Part model, mm, in its own coordinate system. A direction names the side the tool comes from. Give positions to 0.01 mm unless a question says otherwise; leave off trailing zeros. Order: outer loops, then holes, each group sorted by start corner. A loop starts at its lowest first (then second) coordinate and runs counter-clockwise, first axis right, second up.
from build123d import *

# Parameters (mm, degrees)
CROQUIS2_R                          = 7
SALIENTE_EXTRUIR1_DEPTH             = 3
CROQUIS3_R                          = 1.5
SALIENTE_EXTRUIR2_DEPTH             = 6
DI_METRO_DE_TALADRO_3_2_3_2_1_D     = 3.2
DI_METRO_DE_TALADRO_3_2_3_2_1_DEPTH = 10
DI_METRO_DE_TALADRO_4_2_4_2_1_D     = 4.2
DI_METRO_DE_TALADRO_4_2_4_2_1_DEPTH = 12
CHAFL_N1_SIZE                       = 18
CHAFL_N1_SIZE2                      = 4


with BuildPart() as part:
    # Croquis1 → Revolución1 (revolve)
    with BuildSketch(Plane.XY, mode=Mode.PRIVATE) as revoluci_n1_sk:
        with BuildLine():
            Line((34, 38.5), (0, 38.5))
            Line((0, 38.5), (0, 0))
            Line((0, 0), (46, 0))
            Line((46, 0), (46, 30))
            ThreePointArc((46, 30), (41.352720585, 36.159723179), (34, 38.5))
        make_face()
    revolve(revoluci_n1_sk.sketch.rotate(Axis((0, 38.5, 0), (0, -1, 0)), 270), axis=Axis((0, 38.5, 0), (0, -1, 0)))

    # Croquis2 → Saliente-Extruir1 (add)
    with BuildSketch(Plane.XZ):
        with Locations(Location((0, 0, 0), (0, 0, 270))):
            Circle(CROQUIS2_R)
    extrude(amount=SALIENTE_EXTRUIR1_DEPTH)

    # Croquis3 → Saliente-Extruir2 (add)
    with BuildSketch(Plane(origin=(0, 38.5, 0), x_dir=(-1, 0, 0), z_dir=(0, 1, 0))):
        with Locations(Location((0, 0, 0), (0, 0, 90))):
            Circle(CROQUIS3_R)
    extrude(amount=SALIENTE_EXTRUIR2_DEPTH)

    # Diámetro de taladro Ø3.2 (3.2)1
    with Locations(Plane(origin=(0, 38.5, 0), x_dir=(1, 0, 0), z_dir=(0, 1, 0))):
        with Locations((0, 15.5), (-15.5, 0), (15.5, 0), (0, -15.5)):
            Hole(DI_METRO_DE_TALADRO_3_2_3_2_1_D / 2, depth=DI_METRO_DE_TALADRO_3_2_3_2_1_DEPTH)

    # Diámetro de taladro Ø4.2 (4.2)1
    with Locations(Plane(origin=(0, 0, 0), x_dir=(-1, 0, 0), z_dir=(0, -1, 0))):
        with Locations((0, -20), (20, 0), (-20, 0), (0, 20)):
            Hole(DI_METRO_DE_TALADRO_4_2_4_2_1_D / 2, depth=DI_METRO_DE_TALADRO_4_2_4_2_1_DEPTH)

    # Chaflán1
    chafl_n1_edges = [part.edges().sort_by_distance(p)[0] for p in [
        (0, 0, 46),
    ]]
    chafl_n1_side = [part.faces().sort_by_distance(p)[0] for p in [
        (0, 0, 44.698923523),
    ]]
    chamfer(chafl_n1_edges, length=CHAFL_N1_SIZE, length2=CHAFL_N1_SIZE2, reference=chafl_n1_side[0])


solid = part.part
Item 1: Drop flat-ended pins along their axis: P1, Ø2.5, axis at x = 15, z = 0, coming from the +Y side; P2, Ø5, axis at x = -25.5, y = 37, coming from the +Z side; P3, Ø4, axis at y = 20.5, z = -15, coming from the +X side. Give the stop position or say it passes through.
Item 2: Drill centre lines: probe 1 along Y at (x, z) = (-9.5, -15.5); probe 2 along Z at (x, y) = (20, 6); probe 3 along X at (y, z) = (35, -15). Where is each one in solid material? Low to high.
Item 3: Band-saw the part on D-D on y = 24. List the corners of the cut face in (x, z), plus the area to 3 significant figures.
Item 4: Which spindle directions (+Z, -Z, +X, -X, +Y, -Y) get a long thin tool onto all of the face, cutting with end or side? Do faces 5 (the face through (0, 44.5, 0)), 6 (the face through (17.1, 33.43, -0.07)), 7 (the face through (-17.997, 6.084, -0.631)). Say none if no direction does.
Item 5: Band-saw the part on B-B on y = 41.5. List the corners of the cut face in (x, z).
Item 6: Band-saw the part on C-C on y = 34. List the corners of the cut face in (x, z), plus the area to 3 significant figures.
Item 7: Pull direction X, two halves, no side cores. Call faces 1 (the face through (22.003, 6.084, -0.631)), 2 (the face through (0, -3, 0)), 3 (the face through (1.13, 6.08, 18.23)), 4 (the face through (-28.43, 0.25, 6.31)): released by +X, released by -X, zero draft, split by the parting line, or undercut.
Item 8: Band-saw the part on A-A on y = 8. List the corners of the cut face in (x, z).
Working result:
1. P1: stops at y = 38.5
1. P2: stops at z = 35.43
1. P3: stops at x = 44.12
2. probe 1: y = 0 to 38.5
2. probe 2: z = -41.42 to -2.1, 2.1 to 41.42
2. probe 3: x = -40.05 to -1.52, 1.52 to 40.05
3. outline: circle Ø92 at (0, 0)
3. area: 6,650 mm2
4. face 5: +Z, -Z, +X, -X, +Y
4. face 6: +Y
4. face 7: -Y
5. outline: circle Ø3 at (0, 0)
6. outline: circle Ø87.41 at (0, 0); hole circle Ø3.2 at (-15.5, 0); hole circle Ø3.2 at (0, -15.5); hole circle Ø3.2 at (0, 15.5); hole circle Ø3.2 at (15.5, 0)
6. area: 5,970 mm2
7. face 1: undercut
7. face 2: zero draft
7. face 3: undercut
7. face 4: split by the parting line
8. outline: circle Ø92 at (0, 0); hole circle Ø4.2 at (-20, 0); hole circle Ø4.2 at (0, -20); hole circle Ø4.2 at (0, 20); hole circle Ø4.2 at (20, 0)
